```python
from build123d import *

# Parameters (mm, degrees)
CROQUIS1_W                    = 50
CROQUIS1_H                    = 44
SALIENTE_EXTRUIR1_DEPTH       = 1
CROQUIS2_W                    = 50
CROQUIS2_H                    = 1
SALIENTE_EXTRUIR2_DEPTH       = 16
CROQUIS3_W                    = 1
CROQUIS3_H                    = 1
SALIENTE_EXTRUIR3_DEPTH       = 50
CROQUIS4_W                    = 1
CROQUIS4_H                    = 18
SALIENTE_EXTRUIR4_DEPTH       = 1
CROQUIS6_W                    = 1
CROQUIS6_H                    = 18
SALIENTE_EXTRUIR5_DEPTH       = 1
CROQUIS12_W                   = 1
CROQUIS12_H                   = 18
SALIENTE_EXTRUIR11_DEPTH      = 1
CROQUIS13_W                   = 18
CROQUIS13_H                   = 1
SALIENTE_EXTRUIR12_DEPTH      = 21
CROQUIS14_W                   = 18
CROQUIS14_H                   = 1
SALIENTE_EXTRUIR13_DEPTH      = 21
REDONDEO4_R                   = 9
REDONDEO5_R                   = 9
CROQUIS15_W                   = 18
CROQUIS15_H                   = 1
SALIENTE_EXTRUIR14_DEPTH      = 1
CROQUIS16_W                   = 18
CROQUIS16_H                   = 1
SALIENTE_EXTRUIR15_DEPTH      = 1
REDONDEO6_R                   = 5
REDONDEO7_R                   = 5
SALIENTE_EXTRUIR22_DEPTH      = 10
SALIENTE_EXTRUIR22_DEPTH_BACK = 54
CROQUIS17_R                   = 5.5
CORTAR_EXTRUIR5_START         = -2
CROQUIS25_R                   = 5.5
CORTAR_EXTRUIR5_DEPTH         = 2
CROQUIS26_R                   = 4.5
CORTAR_EXTRUIR6_DEPTH         = 97.524608261


# Some blends are built 0.0001 mm under size
with BuildPart() as part:
    # Croquis1 → Saliente-Extruir1 (new body)
    with BuildSketch(Plane.XY):
        with Locations((25, -22)):
            Rectangle(CROQUIS1_W, CROQUIS1_H)
    extrude(amount=SALIENTE_EXTRUIR1_DEPTH)

    # Croquis2 → Saliente-Extruir2 (add)
    with BuildSketch(Plane.XY.offset(1)):
        with Locations((25, -0.5)):
            Rectangle(CROQUIS2_W, CROQUIS2_H)
        with Locations((25, -43.5)):
            Rectangle(CROQUIS2_W, CROQUIS2_H)
    extrude(amount=SALIENTE_EXTRUIR2_DEPTH)

    # Croquis3 → Saliente-Extruir3 (add)
    with BuildSketch(Plane.ZY):
        Polygon((0, -44), (17, -44), (17, -43), (1, -43), (0, -43), align=None)
        with Locations((-0.5, -43.5)):
            Rectangle(CROQUIS3_W, CROQUIS3_H)
        with Locations((-0.5, -0.5)):
            Rectangle(CROQUIS3_W, CROQUIS3_H)
        Polygon((0, 0), (0, -1), (1, -1), (17, -1), (17, 0), align=None)
    extrude(amount=SALIENTE_EXTRUIR3_DEPTH)



with BuildPart() as body_2:
    # Croquis4 → Saliente-Extruir4 (new body)
    with BuildSketch(Plane.XZ.offset(1)):
        with Locations((-50.5, 8)):
            Rectangle(CROQUIS4_W, CROQUIS4_H)
    extrude(amount=SALIENTE_EXTRUIR4_DEPTH)


with BuildPart() as part_1:
    add(part.part)

    add(body_2.part)  # Saliente-Extruir5 merges body 2
    # Croquis6 → Saliente-Extruir5 (add)
    with BuildSketch(Plane(origin=(0, -1, 0), x_dir=(1, 0, 0), z_dir=(0, 1, 0))):
        with Locations((-50.5, -8)):
            Rectangle(CROQUIS6_W, CROQUIS6_H)
    extrude(amount=SALIENTE_EXTRUIR5_DEPTH)

    # Croquis12 → Saliente-Extruir11 (add)
    with BuildSketch(Plane(origin=(0, -43, 0), x_dir=(1, 0, 0), z_dir=(0, 1, 0))):
        with Locations((-49.5, -8)):
            Rectangle(CROQUIS12_W, CROQUIS12_H)
    extrude(amount=SALIENTE_EXTRUIR11_DEPTH)

    # Croquis13 → Saliente-Extruir12 (add)
    with BuildSketch(Plane.ZY.offset(50)):
        with Locations((8, -42.5)):
            Rectangle(CROQUIS13_W, CROQUIS13_H)
    extrude(amount=SALIENTE_EXTRUIR12_DEPTH)

    # Croquis14 → Saliente-Extruir13 (add)
    with BuildSketch(Plane.ZY.offset(51)):
        with Locations((8, -1.5)):
            Rectangle(CROQUIS14_W, CROQUIS14_H)
    extrude(amount=SALIENTE_EXTRUIR13_DEPTH)

    # Redondeo4
    redondeo4_edges = [part_1.edges().sort_by_distance(p)[0] for p in [
        (-72, -1.5, -1),
        (-72, -1.5, 17),
    ]]
    fillet(redondeo4_edges, radius=REDONDEO4_R - 0.0001)  # a hair under: the kernel refuses the full size

    # Redondeo5
    redondeo5_edges = [part_1.edges().sort_by_distance(p)[0] for p in [
        (-71, -42.5, -1),
        (-71, -42.5, 17),
    ]]
    fillet(redondeo5_edges, radius=REDONDEO5_R - 0.0001)  # a hair under: the kernel refuses the full size

    # Croquis15 → Saliente-Extruir14 (add)
    with BuildSketch(Plane(origin=(-49, 0, 0), x_dir=(0, 0, -1), z_dir=(1, 0, 0))):
        with Locations((-8, -42.5)):
            Rectangle(CROQUIS15_W, CROQUIS15_H)
    extrude(amount=SALIENTE_EXTRUIR14_DEPTH)

    # Croquis16 → Saliente-Extruir15 (add)
    with BuildSketch(Plane(origin=(-50, 0, 0), x_dir=(0, 0, -1), z_dir=(1, 0, 0))):
        with Locations((-8, -1.5)):
            Rectangle(CROQUIS16_W, CROQUIS16_H)
    extrude(amount=SALIENTE_EXTRUIR15_DEPTH)

    # Redondeo6
    # the kernel refuses this fillet: 5 mm, written as the material it takes off along each edge
    with BuildSketch(Plane(origin=(-48, -42, -8.5), x_dir=(-1, 0, 0), z_dir=(0, 0, 1))) as redondeo6_piece_1:
        with BuildLine():
            CenterArc((3, 5), REDONDEO6_R, 233.130102354, 36.869897646)
            Line((0, 1), (-0.06, 0.92))
            ThreePointArc((-0.06, 0.92), (-0.1, 0.5), (-0.1, 0))
            Line((-0.1, 0), (0, -0.1))
            Line((0, -0.1), (3, -0.1))
            Line((3, -0.1), (3, 0))
        make_face()
    extrude(amount=33, mode=Mode.SUBTRACT)
    with BuildSketch(Plane(origin=(-49, -2, -8.5), x_dir=(0, 1, 0), z_dir=(0, 0, 1))) as redondeo6_piece_2:
        with BuildLine():
            CenterArc((5, 3), REDONDEO6_R, 180, 36.869897646)
            Line((0, 3), (-0.1, 3))
            Line((-0.1, 3), (-0.1, 0))
            Line((-0.1, 0), (0, -0.1))
            ThreePointArc((0, -0.1), (0.5, -0.1), (0.92, -0.06))
            Line((0.92, -0.06), (1, 0))
        make_face()
    extrude(amount=33, mode=Mode.SUBTRACT)

    # Redondeo7
    # the kernel refuses this fillet: 5 mm, written as the material it takes off along each edge
    with BuildSketch(Plane(origin=(-50, -44, 24.5), x_dir=(1, 0, 0), z_dir=(0, 0, -1)), Plane(origin=(-51, 0, -8.5), x_dir=(1, 0, 0), z_dir=(0, 0, 1))) as redondeo7_piece_1:
        with BuildLine():
            CenterArc((3, -5), REDONDEO7_R, 90, 36.869897646)
            Line((0, -1), (-0.06, -0.92))
            ThreePointArc((-0.06, -0.92), (-0.1, -0.5), (-0.1, 0))
            Line((-0.1, 0), (0, 0.1))
            Line((0, 0.1), (3, 0.1))
            Line((3, 0.1), (3, 0))
        make_face()
    extrude(amount=33, mode=Mode.SUBTRACT)

    # Croquis17 → Saliente-Extruir22 (add, two sides: drawn at the far end of the back side and taken through both)
    with BuildSketch(Plane.XZ.offset(43).offset(-SALIENTE_EXTRUIR22_DEPTH_BACK)):
        with Locations(Location((-62, 8, 0), (0, 0, 270))):
            Circle(CROQUIS17_R)
    extrude(amount=SALIENTE_EXTRUIR22_DEPTH + SALIENTE_EXTRUIR22_DEPTH_BACK)

    # Croquis25 → Cortar-Extruir5 (cut)
    with BuildSketch(Plane(origin=(0, 11, 0), x_dir=(1, 0, 0), z_dir=(0, 1, 0)).offset(CORTAR_EXTRUIR5_START)):
        with Locations(Location((-62, -8, 0), (0, 0, 90))):
            Circle(CROQUIS25_R)
    extrude(amount=CORTAR_EXTRUIR5_DEPTH, mode=Mode.SUBTRACT)

    # Croquis26 → Cortar-Extruir6 (cut, through all)
    with BuildSketch(Plane(origin=(0, 9, 0), x_dir=(1, 0, 0), z_dir=(0, 1, 0))):
        with Locations(Location((-62, -8, 0), (0, 0, 270))):
            Circle(CROQUIS26_R)
    extrude(amount=-CORTAR_EXTRUIR6_DEPTH, mode=Mode.SUBTRACT)


solid = part_1.part
```
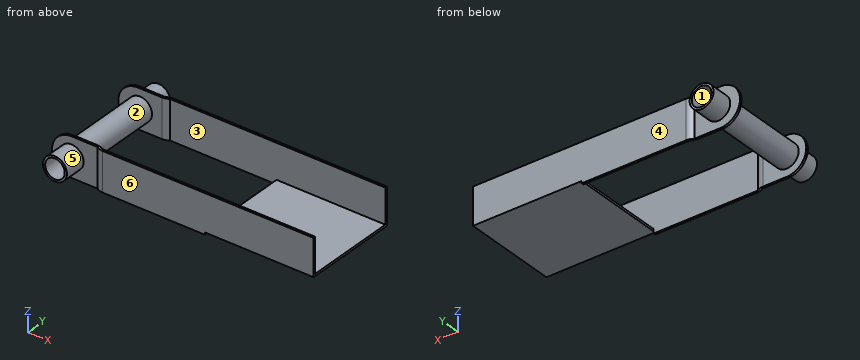
Part model, mm, in its own coordinate system. Face numbers are marked on the shaded views. A direction names the side the tool comes from. Round coordinates to 2 decimals unless told otherwise and drop trailing zeros. Loops run counter-clockwise (first coordinate to the right, second up) from the corner with the lowest first, then second, coordinate; pieces in that order, holes last. Notation, with made-up numbers: (-34, 5) -> (-3, 5) arc R13 cw to (-3, 17) -> close; hole circle Ø1 at (2.5, 39.25). An arc over 180 degrees is marked (long way). Use a Markdown table: item, result.
1) Cut at A-A, the plane x = -4.5. List the corners of the cut face in (y, z), and give its area (3 significant figures).
The answers:
| item | result |
|---|---|
| outline | (-44, -1) -> (-43, -1) -> (-43, 17) -> (-44, 17) -> close; (-1, -1) -> (0, -1) -> (0, 17) -> (-1, 17) -> close |
| area | 36.0 mm2 |
2) Pull direction Z, two halves, no side cores. Call the marked faces 1, 2 and 3: pulls with the +Z half, pulls with the -Z half, needs draft (parallel to the pull), parting line crosses it, or undercut.
The answers:
| item | result |
|---|---|
| face 1 | undercut |
| face 2 | parting line crosses it |
| face 3 | needs draft |
3) Drop flat-ended pins along their axis: pin 1 Ø9 at (x, z) = (12, 4.5) entering from -Y; pin 2 Ø10 at (x, z) = (36.5, 1) entering from +Y; pin 3 Ø4 at (x, y) = (2, -38) entering from +Z; pin 4 Ø5.5 at (x, z) = (-65.5, 10) entering from +Y. Give the stop position or say it passes through.
The answers:
| item | result |
|---|---|
| pin 1 | stops at y = -44 |
| pin 2 | stops at y = 0 |
| pin 3 | stops at z = 1 |
| pin 4 | stops at y = 9 |
4) Cut at D-D, the plane y = 3.5. List the corners of the cut face in (x, z), and give its area (3 significant figures).
The answers:
| item | result |
|---|---|
| outline | circle Ø11 at (-62, 8); hole circle Ø9 at (-62, 8) |
| area | 31.4 mm2 |
5) Probe line 1 (Y direction, x = 12.5, z = 14.25); line 2 (X direction, y = -15, z = 8); line 3 (X direction, y = -42.5, z = 9.5). List the from-to ranges inside material, lowest first. Write a range as [from, to].
The answers:
| item | result |
|---|---|
| line 1 | y = [-44, -43], [-1, 0] |
| line 2 | x = [-67.5, -66.5], [-57.5, -56.5] |
| line 3 | x = [-70.87, -66.24], [-57.76, -48.82] |
6) Cut at B-B, the plane y = -29. List the corners of the cut face in (x, z), and give its area (3 significant figures).
The answers:
| item | result |
|---|---|
| outline | circle Ø11 at (-62, 8); (0, 0) -> (50, 0) -> (50, 1) -> (0, 1) -> close; hole circle Ø9 at (-62, 8) |
| area | 81.4 mm2 |
7) Tool access for the marked faces 4, 5 and 6: list every direction of +Z, -Z, +X, -X, +Y, -Y with a clear straight run to the whole face (end or side of a thin tool).
The answers:
| item | result |
|---|---|
| face 4 | +Z, -Z, +X, +Y |
| face 5 | -Y |
| face 6 | +Z, -Z, +X, -Y |
